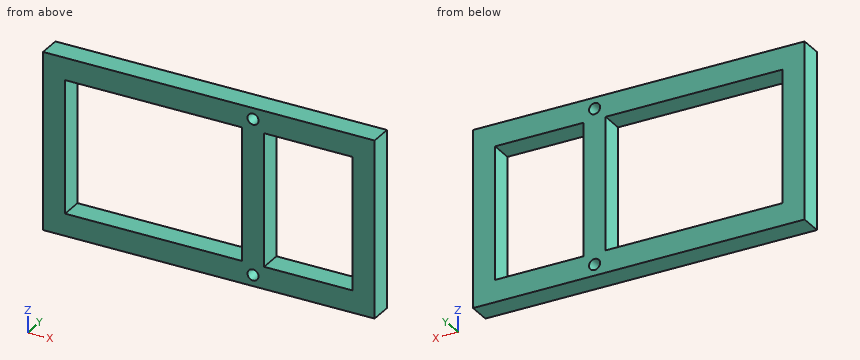
```python
from build123d import *

# Parameters (mm, degrees)
SKETCH1_W           = 150
SKETCH1_H           = 80
BOSS_EXTRUDE1_DEPTH = 10
SKETCH2_W           = 80
SKETCH2_H           = 60
SKETCH2_W_2         = 40
CUT_EXTRUDE1_DEPTH  = 10
SKETCH3_R           = 2.5
CUT_EXTRUDE2_DEPTH  = 86.586213843


with BuildPart() as part:
    # Sketch1 → Boss-Extrude1 (new body)
    with BuildSketch(Plane(origin=(0, 0, 0), x_dir=(1, 0, 0), z_dir=(0, 1, 0))):
        Rectangle(SKETCH1_W, SKETCH1_H)
    extrude(amount=-BOSS_EXTRUDE1_DEPTH)

    # Sketch2 → Cut-Extrude1 (cut)
    with BuildSketch(Plane(origin=(0, 0, 0), x_dir=(1, 0, 0), z_dir=(0, 1, 0))):
        with Locations((-25, 0)):
            Rectangle(SKETCH2_W, SKETCH2_H)
        with Locations((45, 0)):
            Rectangle(SKETCH2_W_2, SKETCH2_H)
    extrude(amount=-CUT_EXTRUDE1_DEPTH, mode=Mode.SUBTRACT)

    # Sketch3 → Cut-Extrude2 (cut, through all)
    with BuildSketch(Plane(origin=(0, 0, 0), x_dir=(1, 0, 0), z_dir=(0, 1, 0))):
        with Locations(Location((20, 35, 0), (0, 0, 270))):
            Circle(SKETCH3_R)
        with Locations(Location((20, -35, 0), (0, 0, 90))):
            Circle(SKETCH3_R)
    extrude(amount=-CUT_EXTRUDE2_DEPTH, mode=Mode.SUBTRACT)


solid = part.part
```
Here's how the part is built. I have some questions about the finished solid (model axes, mm). Coordinates: 2 decimals unless noted, no trailing zeros. Loops run counter-clockwise (first coordinate to the right, second up) from the corner with the lowest first, then second, coordinate; pieces in that order, holes last. Notation, with made-up numbers: (-36, -26.5) - (0, -26.5) arc R18 ccw to (0, -10.5) - close; hole circle Ø8 at (66.5, 38.5). An arc over 180 degrees is marked (long way). Answer as CSV lines item,"result".
Q1. If we section it at B-B, the plane x = 20: Write out the boundary of the cut face in (y, z).
Response:
outline,"(-10, -40) - (0, -40) - (0, -37.5) - (-10, -37.5) - close; (-10, -32.5) - (0, -32.5) - (0, 32.5) - (-10, 32.5) - close; (-10, 37.5) - (0, 37.5) - (0, 40) - (-10, 40) - close"
Q2. If we section it at D-D, the plane x = -19: Write out the boundary of the cut face in (y, z), and give its area (3 significant figures).
Response:
outline,"(-10, -40) - (0, -40) - (0, -30) - (-10, -30) - close; (-10, 30) - (0, 30) - (0, 40) - (-10, 40) - close"
area,"200 mm2"
Q3. If I drill on L1, parallel to X at y = -4.75, z = 11.5; L2, parallel to X at y = -2.5, z = -35; L3, parallel to Z at x = 0, y = -1.5, over which ranges is the centre line in solid material (lowest first)? Write a range as [from, to].
Response:
L1,"[-75, -65], [15, 25], [65, 75]"
L2,"[-75, 17.5], [22.5, 75]"
L3,"[-40, -30], [30, 40]"
Q4. If we section it at A-A, the plane z = 21: Write out the boundary of the cut face in (x, y), and give its area (3 significant figures).
Response:
outline,"(-75, -10) - (-65, -10) - (-65, 0) - (-75, 0) - close; (15, -10) - (25, -10) - (25, 0) - (15, 0) - close; (65, -10) - (75, -10) - (75, 0) - (65, 0) - close"
area,"300 mm2"
Q5. If we section it at C-C, the plane z = -35: Write out the boundary of the cut face in (x, y).
Response:
outline,"(-75, -10) - (17.5, -10) - (17.5, 0) - (-75, 0) - close; (22.5, -10) - (75, -10) - (75, 0) - (22.5, 0) - close"
